Source: three-view drawing plus pictorial views. Frame: mm from the lowest corner of the part. A direction names the side the tool comes from. Give positions to 0.01 mm unless a question says otherwise; leave off trailing zeros. Order: outer loops, then holes, each group sorted by start corner. A loop starts at its lowest first (then second) coordinate and runs counter-clockwise, first axis right, second up. Notation, with made-up numbers: (22, -19) -> (34, -19) arc R19 ccw to (34, -8) -> close; hole circle Ø6 at (43, 32). An arc over 180 degrees is marked (long way). Write item = value, one per line.
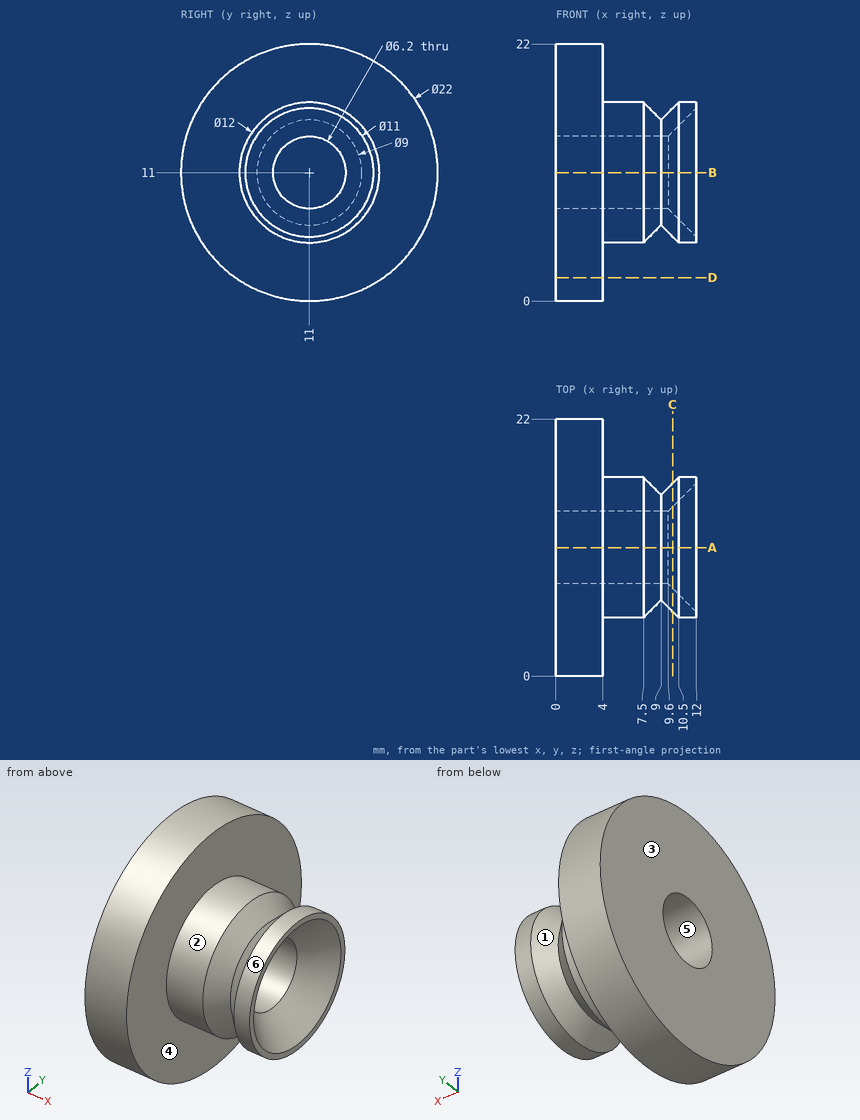
1) First-contact query: P1, Ø1, axis at x = 3.5, z = 6, coming from the +Y side; P2, Ø4, axis at x = 7, z = 13.5, coming from the -Y side; P3, Ø3, axis at x = 10.5, z = 12, coming from the +Y side. Flat tips, straight axial feed; report the tip coordinate or a pass-through.
Check sheet entries:
P1 = 21.04
P2 = 5.02
P3 = 17
2) Section query C-C (x = 10). Output: boundary loops of the cut face in (y, z).
Check sheet entries:
outline = circle Ø11 at (11, 11); hole circle Ø7 at (11, 11)
3) Mould query, pull axis Z, two halves, no side actions, for the marked faces 4, 5 and 6. Classes: +Z half, -Z half, draft (parallel to the pull), parting line (faces both ways), or undercut.
Check sheet entries:
face_4 = draft
face_5 = undercut
face_6 = parting line
4) Section query A-A (y = 11). Output: boundary loops of the cut face in (x, z), plus the area to 3 significant figures.
Check sheet entries:
outline = (0, 0) -> (4, 0) -> (4, 5) -> (7.5, 5) -> (9, 6.5) -> (10.5, 5) -> (12, 5) -> (12, 5.5) -> (9.6, 7.9) -> (0, 7.9) -> close; (0, 14.1) -> (9.6, 14.1) -> (12, 16.5) -> (12, 17) -> (10.5, 17) -> (9, 15.5) -> (7.5, 17) -> (4, 17) -> (4, 22) -> (0, 22) -> close
area = 99.3 mm²
5) Reachability of the marked faces 1, 2 and 3 from +Z, -Z, +X, -X, +Y, -Y: full face, straight path, thin tool, end or side. Return the list, or none.
Check sheet entries:
face_1 = none
face_2 = +X
face_3 = +Z, -Z, -X, +Y, -Y
6) Section query D-D (z = 2). Output: boundary loops of the cut face in (x, y), plus the area to 3 significant figures.
Check sheet entries:
outline = (0, 4.68) -> (4, 4.68) -> (4, 17.32) -> (0, 17.32) -> close
area = 50.6 mm²
7) Line query: line 1 (Z direction, x = 6.25, y = 11); line 2 (Z direction, x = 3.75, y = 11); line 3 (X direction, y = 3.75, z = 10). Output: solid intervals per line, ascending. Write a range as from..to.
Check sheet entries:
line_1 = 5..7.9, 14.1..17
line_2 = 0..7.9, 14.1..22
line_3 = 0..4
